Could you check a few things on this model? Use its own coordinates, in mm. Face numbers are marked on the shaded views. Give positions to 0.01 mm unless a question says otherwise; leave off trailing zeros. Loops run counter-clockwise (first coordinate to the right, second up) from the corner with the lowest first, then second, coordinate; pieces in that order, holes last. Notation, with made-up numbers: M 57.5,68.5 L 85.5,68.5 A13 ccw 85.5,81.5 Z; hole C 52.5,80.5 d6. An arc over 180 degrees is marked long. Return JSON: item names as keys, results as strings. Group by question number.
1. Please list where these lines run through material, in increasing order: line 1 (Y direction, x = 19, z = 7.25); line 2 (X direction, y = 12, z = 1.5); line 3 (Z direction, x = -19.5, y = 6).
2. If we section it at B-B (z = 6.75): State how many separate pieces and enclosed holes the cut face has, plus the area to 3 significant figures.
3. For pin 1 (5 mm diameter, centred on x = -45, y = 0, fed in from +Z); pin 2 (6 mm diameter, centred on y = -33.5, z = 6, fed in from +X); pin 3 (2.5 mm diameter, centred on x = -31.82, y = 31.82, fed in from +Z), each with a flat end and sliding along its axis, tell me the tip position at first contact or that it passes through.
4. If we section it at A-A (x = 0): Write out the boundary of the cut face in (y, z) (3 decimals), plus the area to 3 significant figures.
5. If we mould it in two halves opening along Y, with no side actions, what happens to the marked faces 1, 2 and 3? For each: +Y half, -Y half, draft (parallel to the pull), parting line (faces both ways), or undercut.
```python
from build123d import *

# Parameters (mm, degrees)
SKETCH3_R           = 59.5
BOSS_EXTRUDE1_DEPTH = 10
SKETCH4_R           = 1.6
CUT_EXTRUDE1_DEPTH  = 85.737830985
SKETCH5_R           = 2
CUT_EXTRUDE2_DEPTH  = 5
SKETCH6_R           = 2.9
CUT_EXTRUDE3_DEPTH  = 3
SKETCH7_R           = 23.435
CUT_EXTRUDE4_DEPTH  = 7
SKETCH8_R           = 20.25
CUT_EXTRUDE5_DEPTH  = 85.737830985
CHAMFER1_SIZE       = 1.2


with BuildPart() as part:
    # Sketch3 → Boss-Extrude1 (new body)
    with BuildSketch(Plane.XY):
        Circle(SKETCH3_R)
    extrude(amount=BOSS_EXTRUDE1_DEPTH)

    # Sketch4 → Cut-Extrude1 (cut, through all)
    with BuildSketch(Plane.XY.offset(10)):
        with Locations((44.782953319, 29.92301275)):
            Circle(SKETCH4_R)
        with Locations((52.825095203, -10.507564744)):
            Circle(SKETCH4_R)
        with Locations((29.92301275, -44.782953319)):
            Circle(SKETCH4_R)
        with Locations((-10.507564744, -52.825095203)):
            Circle(SKETCH4_R)
        with Locations((-44.782953319, -29.92301275)):
            Circle(SKETCH4_R)
        with Locations((-52.825095203, 10.507564744)):
            Circle(SKETCH4_R)
        with Locations((-29.92301275, 44.782953319)):
            Circle(SKETCH4_R)
        with Locations((10.507564744, 52.825095203)):
            Circle(SKETCH4_R)
    extrude(amount=-CUT_EXTRUDE1_DEPTH, mode=Mode.SUBTRACT)

    # Sketch5 → Cut-Extrude2 (cut)
    with BuildSketch(Plane.XY.offset(10)):
        with Locations((45, 0)):
            Circle(SKETCH5_R)
        with Locations((41.574578963, -17.220754456)):
            Circle(SKETCH5_R)
        with Locations((31.819805153, -31.819805153)):
            Circle(SKETCH5_R)
        with Locations((17.220754456, -41.574578963)):
            Circle(SKETCH5_R)
        with Locations((0, -45)):
            Circle(SKETCH5_R)
        with Locations((-17.220754456, -41.574578963)):
            Circle(SKETCH5_R)
        with Locations((-31.819805153, -31.819805153)):
            Circle(SKETCH5_R)
        with Locations((-41.574578963, -17.220754456)):
            Circle(SKETCH5_R)
        with Locations((-45, 0)):
            Circle(SKETCH5_R)
        with Locations((-41.574578963, 17.220754456)):
            Circle(SKETCH5_R)
        with Locations((-31.819805153, 31.819805153)):
            Circle(SKETCH5_R)
        with Locations((-17.220754456, 41.574578963)):
            Circle(SKETCH5_R)
        with Locations((0, 45)):
            Circle(SKETCH5_R)
        with Locations((17.220754456, 41.574578963)):
            Circle(SKETCH5_R)
        with Locations((31.819805153, 31.819805153)):
            Circle(SKETCH5_R)
        with Locations((41.574578963, 17.220754456)):
            Circle(SKETCH5_R)
    extrude(amount=-CUT_EXTRUDE2_DEPTH, mode=Mode.SUBTRACT)

    # Sketch6 → Cut-Extrude3 (cut)
    with BuildSketch(Plane(origin=(0, 0, 0), x_dir=(-1, 0, 0), z_dir=(0, 0, -1))):
        with Locations((52.825095203, 10.507564744)):
            Circle(SKETCH6_R)
        with Locations((44.782953319, -29.92301275)):
            Circle(SKETCH6_R)
        with Locations((10.507564744, -52.825095203)):
            Circle(SKETCH6_R)
        with Locations((-29.92301275, -44.782953319)):
            Circle(SKETCH6_R)
        with Locations((-52.825095203, -10.507564744)):
            Circle(SKETCH6_R)
        with Locations((-44.782953319, 29.92301275)):
            Circle(SKETCH6_R)
        with Locations((-10.507564744, 52.825095203)):
            Circle(SKETCH6_R)
        with Locations((29.92301275, 44.782953319)):
            Circle(SKETCH6_R)
    extrude(amount=-CUT_EXTRUDE3_DEPTH, mode=Mode.SUBTRACT)

    # Sketch7 → Cut-Extrude4 (cut)
    with BuildSketch(Plane.XY.offset(10)):
        Circle(SKETCH7_R)
    extrude(amount=-CUT_EXTRUDE4_DEPTH, mode=Mode.SUBTRACT)

    # Sketch8 → Cut-Extrude5 (cut, through all)
    with BuildSketch(Plane.XY.offset(10)):
        Circle(SKETCH8_R)
    extrude(amount=-CUT_EXTRUDE5_DEPTH, mode=Mode.SUBTRACT)

    # Chamfer1
    chamfer1_edges = [part.edges().sort_by_distance(p)[0] for p in [
        (39.574578963, 17.220754456, 10),
        (29.819805153, 31.819805153, 10),
        (15.220754456, 41.574578963, 10),
        (-2, 45, 10),
        (-19.220754456, 41.574578963, 10),
        (-33.819805153, 31.819805153, 10),
        (-43.574578963, 17.220754456, 10),
        (-47, 0, 10),
        (-43.574578963, -17.220754456, 10),
        (-33.819805153, -31.819805153, 10),
        (-19.220754456, -41.574578963, 10),
        (-2, -45, 10),
        (15.220754456, -41.574578963, 10),
        (29.819805153, -31.819805153, 10),
        (39.574578963, -17.220754456, 10),
        (43, 0, 10),
    ]]
    chamfer(chamfer1_edges, length=CHAMFER1_SIZE)


solid = part.part
```
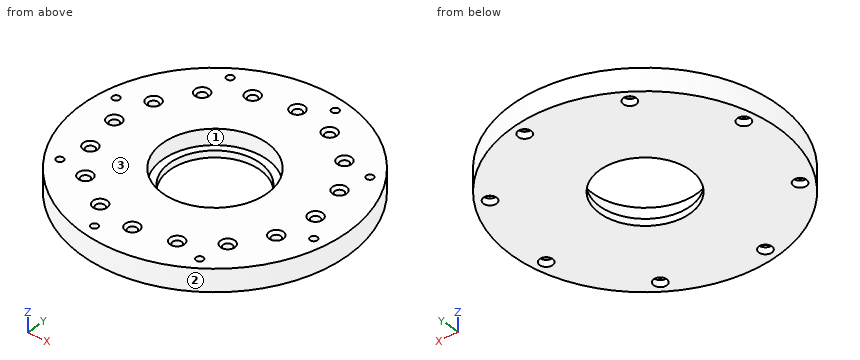
Answer:
{
 "1": {"line 1": "y = -56.38 to -42.49, -40.66 to -13.72, 13.72 to 40.66, 42.49 to 56.38", "line 2": "x = -58.28 to -55.31, -50.34 to -16.31, 16.31 to 58.28", "line 3": "z = 0 to 3"},
 "2": {"separate pieces": "1", "enclosed holes": "25", "area": "9,130 mm²"},
 "3": {"pin 1": "stops at z = 9.3", "pin 2": "stops at x = 51.09", "pin 3": "stops at z = 5"},
 "4": {"outline": "M -59.5,0 L -20.25,0 L -20.25,3 L -23.435,3 L -23.435,10 L -41.8,10 L -43,8.8 L -43,5 L -47,5 L -47,8.8 L -48.2,10 L -59.5,10 Z; M 20.25,0 L 59.5,0 L 59.5,10 L 48.2,10 L 47,8.8 L 47,5 L 43,5 L 43,8.8 L 41.8,10 L 23.435,10 L 23.435,3 L 20.25,3 Z", "area": "698 mm²"},
 "5": {"face 1": "undercut", "face 2": "parting line", "face 3": "draft"}
}
